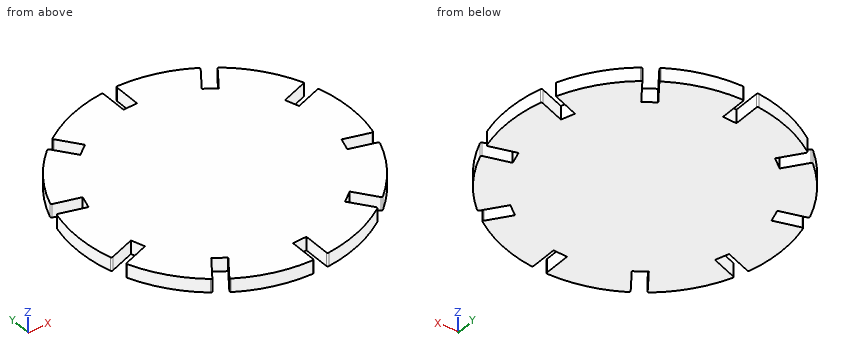
from build123d import *

# Parameters (mm, degrees)
F1_DEPTH = 5


with BuildPart() as f1:
    # F0 (on Top) → F1 (new body)
    with BuildSketch(Plane.XY):
        with BuildLine():
            ThreePointArc((-31.045091, 38.519181), (-31.386265, 38.721261), (-31.767273, 38.611402))
            ThreePointArc((-31.767273, 38.611402), (-40.45085, 29.389263), (-46.538253, 18.280892))
            ThreePointArc((-46.538253, 18.280892), (-46.524997, 17.884584), (-46.227379, 17.622555))
            Line((-46.227379, 17.622555), (-37.277444, 14.714545))
            Line((-37.277444, 14.714545), (-38.807078, 10.006815))
            Line((-38.807078, 10.006815), (-47.757013, 12.914825))
            ThreePointArc((-47.757013, 12.914825), (-48.151808, 12.877774), (-48.395476, 12.564946))
            ThreePointArc((-48.395476, 12.564946), (-50, 0), (-48.395476, -12.564946))
            ThreePointArc((-48.395476, -12.564946), (-48.151808, -12.877774), (-47.757013, -12.914825))
            Line((-47.757013, -12.914825), (-38.807078, -10.006815))
            Line((-38.807078, -10.006815), (-37.277444, -14.714545))
            Line((-37.277444, -14.714545), (-46.227379, -17.622555))
            ThreePointArc((-46.227379, -17.622555), (-46.524997, -17.884584), (-46.538253, -18.280892))
            ThreePointArc((-46.538253, -18.280892), (-40.45085, -29.389263), (-31.767273, -38.611402))
            ThreePointArc((-31.767273, -38.611402), (-31.386265, -38.721261), (-31.045091, -38.519181))
            Line((-31.045091, -38.519181), (-25.513727, -30.905911))
            Line((-25.513727, -30.905911), (-21.509093, -33.815448))
            Line((-21.509093, -33.815448), (-27.040457, -41.428718))
            ThreePointArc((-27.040457, -41.428718), (-27.127218, -41.815639), (-26.904999, -42.144051))
            ThreePointArc((-26.904999, -42.144051), (-15.45085, -47.552826), (-3.005051, -49.909615))
            ThreePointArc((-3.005051, -49.909615), (-2.632236, -49.774542), (-2.475, -49.410519))
            Line((-2.475, -49.410519), (-2.475, -40))
            Line((-2.475, -40), (2.475, -40))
            Line((2.475, -40), (2.475, -49.410519))
            ThreePointArc((2.475, -49.410519), (2.632236, -49.774542), (3.005051, -49.909615))
            ThreePointArc((3.005051, -49.909615), (15.45085, -47.552826), (26.904999, -42.144051))
            ThreePointArc((26.904999, -42.144051), (27.127218, -41.815639), (27.040457, -41.428718))
            Line((27.040457, -41.428718), (21.509093, -33.815448))
            Line((21.509093, -33.815448), (25.513727, -30.905911))
            Line((25.513727, -30.905911), (31.045091, -38.519181))
            ThreePointArc((31.045091, -38.519181), (31.386265, -38.721261), (31.767273, -38.611402))
            ThreePointArc((31.767273, -38.611402), (40.45085, -29.389263), (46.538253, -18.280892))
            ThreePointArc((46.538253, -18.280892), (46.524997, -17.884584), (46.227379, -17.622555))
            Line((46.227379, -17.622555), (37.277444, -14.714545))
            Line((37.277444, -14.714545), (38.807078, -10.006815))
            Line((38.807078, -10.006815), (47.757013, -12.914825))
            ThreePointArc((47.757013, -12.914825), (48.151808, -12.877774), (48.395476, -12.564946))
            ThreePointArc((48.395476, -12.564946), (50, 0), (48.395476, 12.564946))
            ThreePointArc((48.395476, 12.564946), (48.151808, 12.877774), (47.757013, 12.914825))
            Line((47.757013, 12.914825), (38.807078, 10.006815))
            Line((38.807078, 10.006815), (37.277444, 14.714545))
            Line((37.277444, 14.714545), (46.729715, 17.785774))
            ThreePointArc((46.729715, 17.785774), (40.606292, 29.174116), (31.767273, 38.611402))
            ThreePointArc((31.767273, 38.611402), (31.386265, 38.721261), (31.045091, 38.519181))
            Line((31.045091, 38.519181), (25.513727, 30.905911))
            Line((25.513727, 30.905911), (21.509093, 33.815448))
            Line((21.509093, 33.815448), (27.040457, 41.428718))
            ThreePointArc((27.040457, 41.428718), (27.127218, 41.815639), (26.904999, 42.144051))
            ThreePointArc((26.904999, 42.144051), (15.45085, 47.552826), (3.005051, 49.909615))
            ThreePointArc((3.005051, 49.909615), (2.632236, 49.774542), (2.475, 49.410519))
            Line((2.475, 49.410519), (2.475, 40))
            Line((2.475, 40), (-2.475, 40))
            Line((-2.475, 40), (-2.475, 49.410519))
            ThreePointArc((-2.475, 49.410519), (-2.632236, 49.774542), (-3.005051, 49.909615))
            ThreePointArc((-3.005051, 49.909615), (-15.45085, 47.552826), (-26.904999, 42.144051))
            ThreePointArc((-26.904999, 42.144051), (-27.127218, 41.815639), (-27.040457, 41.428718))
            Line((-27.040457, 41.428718), (-21.509093, 33.815448))
            Line((-21.509093, 33.815448), (-25.513727, 30.905911))
            Line((-25.513727, 30.905911), (-31.045091, 38.519181))
        make_face()
    extrude(amount=F1_DEPTH)


solid = f1.part
Source: CAD feature listing. Evaluate the final solid. Frame: model axes, mm. Round coordinates to 2 decimals unless told otherwise and drop trailing zeros. Order: outer loops, then holes, each group sorted by start corner. A loop starts at its lowest first (then second) coordinate and runs counter-clockwise, first axis right, second up. Notation, with made-up numbers: (88, -33.5) - (121, -33.5) arc R17 cw to (121, -2.5) - close; hole circle Ø2 at (45.5, 89). An arc over 180 degrees is marked (long way). Use a Markdown table: item, result. Add a question column.
1. Section query B-B (y = -25). Return the cut outline in (x, z).
2. First-contact query: pin 1 (1.5 mm diameter, centred on y = 46, z = 2, fed in from -X); pin 2 (1.5 mm diameter, centred on y = -43, z = 2.5, fed in from -X); pin 3 (3 mm diameter, centred on x = -33.5, y = -2.5, fed in from -Z); pin 4 (1.5 mm diameter, centred on y = -47, z = 2.5, fed in from +X). Flat tips, straight axial feed; report the tip coordinate or a pass-through.
3. Section query A-A (x = 43.5). Return the cut outline in (y, z), then the cut area to 3 significant figures.
4. Line query: probe 1 along X at (y, z) = (-36, 0.65); probe 2 along Y at (x, z) = (39, 4.7); probe 3 along X at (y, z) = (36.5, 0.55). Output: solid intervals per line, ascending.
5. Section query C-C (x = 17.5). Return the cut outline in (y, z), then the cut area to 3 significant figures.
Derived:
| question | item | result |
|---|---|---|
| 1 | outline | (-43.3, 0) - (43.3, 0) - (43.3, 5) - (-43.3, 5) - close |
| 2 | pin 1 | x = -21.27 |
| 2 | pin 2 | x = -26.74 |
| 2 | pin 3 | z = 0 |
| 2 | pin 4 | x = 19 |
| 3 | outline | (-24.65, 0) - (-16.74, 0) - (-16.74, 5) - (-24.65, 5) - close; (-11.53, 0) - (11.53, 0) - (11.53, 5) - (-11.53, 5) - close; (16.74, 0) - (24.65, 0) - (24.65, 5) - (16.74, 5) - close |
| 3 | area | 194 mm2 |
| 4 | probe 1 | -34.7 to -29.21, -23.1 to 23.1, 29.21 to 34.7 |
| 4 | probe 2 | -31.29 to -15.27, -10.07 to 10.07, 15.27 to 31.29 |
| 4 | probe 3 | -34.17 to -29.58, -23.46 to 23.46, 29.58 to 34.17 |
| 5 | outline | (-46.84, 0) - (46.84, 0) - (46.84, 5) - (-46.84, 5) - close |
| 5 | area | 468 mm2 |
